```python
from build123d import *

# Parameters (mm, degrees)
BOSS_EXTRU_1_DEPTH = 150
CONG_1_R           = 15
BOSS_EXTRU_2_DEPTH = 2


with BuildPart() as part:
    # Esquisse1 → Boss.-Extru.1 (new body)
    with BuildSketch(Plane.XY):
        with BuildLine():
            Line((-112.5, 0), (112.5, 0))
            Line((112.5, 0), (112.5, 77.803254504))
            ThreePointArc((112.5, 77.803254504), (109.706079374, 82.982099708), (103.843702056, 83.490983093))
            Line((103.843702056, 83.490983093), (100.822174185, 82.206822173))
            Line((100.822174185, 82.206822173), (101.593849269, 84))
            Line((101.593849269, 84), (100.593849269, 84))
            Line((100.593849269, 84), (98.047294459, 81.066628108))
            Line((98.047294459, 81.066628108), (94.513975375, 79.668180307))
            Line((94.513975375, 79.668180307), (96.868414967, 84))
            Line((96.868414967, 84), (95.868414967, 84))
            Line((95.868414967, 84), (91.710401321, 78.600485349))
            Line((91.710401321, 78.600485349), (88.141932533, 77.29433432))
            Line((88.141932533, 77.29433432), (91.793248094, 84))
            Line((91.793248094, 84), (90.793248094, 84))
            Line((90.793248094, 84), (85.311557961, 76.299859694))
            Line((85.311557961, 76.299859694), (81.710349964, 75.086887739))
            Line((81.710349964, 75.086887739), (86.372418591, 84))
            Line((86.372418591, 84), (85.372418591, 84))
            Line((85.372418591, 84), (78.855086787, 74.166305212))
            Line((78.855086787, 74.166305212), (75.223572191, 73.047331693))
            Line((75.223572191, 73.047331693), (80.613241264, 84))
            Line((80.613241264, 84), (79.613241264, 84))
            Line((79.613241264, 84), (72.345349134, 72.201263116))
            Line((72.345349134, 72.201263116), (68.685981021, 71.177043896))
            Line((68.685981021, 71.177043896), (74.526463538, 84))
            Line((74.526463538, 84), (73.526463538, 84))
            Line((73.526463538, 84), (65.786742319, 70.406060788))
            Line((65.786742319, 70.406060788), (62.101992586, 69.477287727))
            Line((62.101992586, 69.477287727), (68.126397614, 84))
            Line((68.126397614, 84), (67.126397614, 84))
            Line((67.126397614, 84), (59.183696671, 68.781910885))
            Line((59.183696671, 68.781910885), (55.476054359, 67.949211366))
            Line((55.476054359, 67.949211366), (61.430986278, 84))
            Line((61.430986278, 84), (60.430986278, 84))
            Line((60.430986278, 84), (52.540672534, 67.329910517))
            Line((52.540672534, 67.329910517), (48.81264215, 66.593847028))
            Line((48.81264215, 66.593847028), (54.461792967, 84))
            Line((54.461792967, 84), (53.461792967, 84))
            Line((53.461792967, 84), (45.862157261, 66.051040507))
            Line((45.862157261, 66.051040507), (42.116257084, 65.412110258))
            Line((42.116257084, 65.412110258), (47.243908802, 84))
            Line((47.243908802, 84), (46.243908802, 84))
            Line((46.243908802, 84), (39.152662178, 64.946164731))
            Line((39.152662178, 64.946164731), (35.391422557, 64.404799318))
            Line((35.391422557, 64.404799318), (39.805772012, 84))
            Line((39.805772012, 84), (38.805772012, 84))
            Line((38.805772012, 84), (32.416719538, 64.01602953))
            Line((32.416719538, 64.01602953), (28.642681183, 63.572594644))
            Line((28.642681183, 63.572594644), (32.178898512, 84))
            Line((32.178898512, 84), (31.178898512, 84))
            Line((31.178898512, 84), (25.658879458, 63.261263209))
            Line((25.658879458, 63.261263209), (21.874591726, 62.91605839))
            Line((21.874591726, 62.91605839), (24.397526133, 84))
            Line((24.397526133, 84), (23.397526133, 84))
            Line((23.397526133, 84), (18.883706848, 62.682375611))
            Line((18.883706848, 62.682375611), (15.09172602, 62.435634044))
            Line((15.09172602, 62.435634044), (16.498178932, 84))
            Line((16.498178932, 84), (15.498178932, 84))
            Line((15.498178932, 84), (12.095778325, 62.279757774))
            Line((12.095778325, 62.279757774), (8.298665877, 62.131646133))
            Line((8.298665877, 62.131646133), (8.519161913, 84))
            Line((8.519161913, 84), (7.519161913, 84))
            Line((7.519161913, 84), (5.299679125, 62.053681665))
            Line((5.299679125, 62.053681665), (1.5, 62.004299999))
            Line((1.5, 62.004299999), (1, 84))
            Line((1, 84), (-1, 84))
            Line((-1, 84), (-1.5, 62.004299999))
            Line((-1.5, 62.004299999), (-5.299679125, 62.053681665))
            Line((-5.299679125, 62.053681665), (-7.519161913, 84))
            Line((-7.519161913, 84), (-8.519161913, 84))
            Line((-8.519161913, 84), (-8.298665877, 62.131646133))
            Line((-8.298665877, 62.131646133), (-12.095778325, 62.279757774))
            Line((-12.095778325, 62.279757774), (-15.498178932, 84))
            Line((-15.498178932, 84), (-16.498178932, 84))
            Line((-16.498178932, 84), (-15.09172602, 62.435634044))
            Line((-15.09172602, 62.435634044), (-18.883706848, 62.682375611))
            Line((-18.883706848, 62.682375611), (-23.397526133, 84))
            Line((-23.397526133, 84), (-24.397526133, 84))
            Line((-24.397526133, 84), (-21.874591726, 62.91605839))
            Line((-21.874591726, 62.91605839), (-25.658879458, 63.261263209))
            Line((-25.658879458, 63.261263209), (-31.178898512, 84))
            Line((-31.178898512, 84), (-32.178898512, 84))
            Line((-32.178898512, 84), (-28.642681183, 63.572594644))
            Line((-28.642681183, 63.572594644), (-32.416719538, 64.01602953))
            Line((-32.416719538, 64.01602953), (-38.805772012, 84))
            Line((-38.805772012, 84), (-39.805772012, 84))
            Line((-39.805772012, 84), (-35.391422557, 64.404799318))
            Line((-35.391422557, 64.404799318), (-39.152662178, 64.946164731))
            Line((-39.152662178, 64.946164731), (-46.243908802, 84))
            Line((-46.243908802, 84), (-47.243908802, 84))
            Line((-47.243908802, 84), (-42.116257084, 65.412110258))
            Line((-42.116257084, 65.412110258), (-45.862157261, 66.051040507))
            Line((-45.862157261, 66.051040507), (-53.461792967, 84))
            Line((-53.461792967, 84), (-54.461792967, 84))
            Line((-54.461792967, 84), (-48.81264215, 66.593847028))
            Line((-48.81264215, 66.593847028), (-52.540672534, 67.329910517))
            Line((-52.540672534, 67.329910517), (-60.430986278, 84))
            Line((-60.430986278, 84), (-61.430986278, 84))
            Line((-61.430986278, 84), (-55.476054359, 67.949211366))
            Line((-55.476054359, 67.949211366), (-59.183696671, 68.781910885))
            Line((-59.183696671, 68.781910885), (-67.126397614, 84))
            Line((-67.126397614, 84), (-68.126397614, 84))
            Line((-68.126397614, 84), (-62.101992586, 69.477287727))
            Line((-62.101992586, 69.477287727), (-65.786742319, 70.406060788))
            Line((-65.786742319, 70.406060788), (-73.526463538, 84))
            Line((-73.526463538, 84), (-74.526463538, 84))
            Line((-74.526463538, 84), (-68.685981021, 71.177043896))
            Line((-68.685981021, 71.177043896), (-72.345349134, 72.201263116))
            Line((-72.345349134, 72.201263116), (-79.613241264, 84))
            Line((-79.613241264, 84), (-80.613241264, 84))
            Line((-80.613241264, 84), (-75.223572191, 73.047331693))
            Line((-75.223572191, 73.047331693), (-78.855086787, 74.166305212))
            Line((-78.855086787, 74.166305212), (-85.372418591, 84))
            Line((-85.372418591, 84), (-86.372418591, 84))
            Line((-86.372418591, 84), (-81.710349964, 75.086887739))
            Line((-81.710349964, 75.086887739), (-85.311557961, 76.299859694))
            Line((-85.311557961, 76.299859694), (-90.793248094, 84))
            Line((-90.793248094, 84), (-91.793248094, 84))
            Line((-91.793248094, 84), (-88.141932533, 77.29433432))
            Line((-88.141932533, 77.29433432), (-91.710401321, 78.600485349))
            Line((-91.710401321, 78.600485349), (-95.868414967, 84))
            Line((-95.868414967, 84), (-96.868414967, 84))
            Line((-96.868414967, 84), (-94.513975375, 79.668180307))
            Line((-94.513975375, 79.668180307), (-98.047294459, 81.066628108))
            Line((-98.047294459, 81.066628108), (-100.593849269, 84))
            Line((-100.593849269, 84), (-101.593849269, 84))
            Line((-101.593849269, 84), (-100.822174185, 82.206822173))
            Line((-100.822174185, 82.206822173), (-103.843702056, 83.490983093))
            ThreePointArc((-103.843702056, 83.490983093), (-109.706079374, 82.982099708), (-112.5, 77.803254504))
            Line((-112.5, 77.803254504), (-112.5, 0))
        make_face()
    extrude(amount=BOSS_EXTRU_1_DEPTH)

    # Congé1
    cong_1_edges = [part.edges().sort_by_distance(p)[0] for p in [
        (112.5, 0, 75),
        (-112.5, 0, 75),
    ]]
    fillet(cong_1_edges, radius=CONG_1_R)

    # Esquisse2 → Boss.-Extru.2 (add)
    # profile 1 of 2: a face of its own
    with BuildSketch(Plane.XZ):
        Polygon((85, 134), (111, 150), (125, 150), (125, 102), (99, 86), (99, 64), (125, 48), (125, 0), (111, 0), (85, 16), (85, 34.748316978), align=None)
        with BuildLine():
            Line((120.5, 133), (120.5, 117))
            ThreePointArc((120.5, 117), (118.5, 115), (116.5, 117))
            Line((116.5, 117), (116.5, 133))
            ThreePointArc((116.5, 133), (118.5, 135), (120.5, 133))
        make_face(mode=Mode.SUBTRACT)
        with BuildLine():
            Line((120.5, 17), (120.5, 33))
            ThreePointArc((120.5, 33), (118.5, 35), (116.5, 33))
            Line((116.5, 33), (116.5, 17))
            ThreePointArc((116.5, 17), (118.5, 15), (120.5, 17))
        make_face(mode=Mode.SUBTRACT)
    # profile 2 of 2: a face of its own
    with BuildSketch(Plane.XZ):
        Polygon((-85, 34.748316978), (-85, 134), (-111, 150), (-125, 150), (-125, 102), (-99, 86), (-99, 64), (-125, 48), (-125, 0), (-111, 0), (-85, 16), align=None)
        with BuildLine():
            Line((-120.5, 133), (-120.5, 117))
            ThreePointArc((-120.5, 117), (-118.5, 115), (-116.5, 117))
            Line((-116.5, 117), (-116.5, 133))
            ThreePointArc((-116.5, 133), (-118.5, 135), (-120.5, 133))
        make_face(mode=Mode.SUBTRACT)
        with BuildLine():
            Line((-120.5, 17), (-120.5, 33))
            ThreePointArc((-120.5, 33), (-118.5, 35), (-116.5, 33))
            Line((-116.5, 33), (-116.5, 17))
            ThreePointArc((-116.5, 17), (-118.5, 15), (-120.5, 17))
        make_face(mode=Mode.SUBTRACT)
    extrude(amount=BOSS_EXTRU_2_DEPTH)


solid = part.part
```
The listing builds one solid part. Answer for the finished solid, in the listing's coordinates (mm). A direction names the side the tool comes from. Coordinates: 2 decimals unless noted, no trailing zeros. Write each loop counter-clockwise with the first axis right and the second up, starting at its lowest first coordinate (ties: lowest second). Pieces come first, ordered by that corner, then holes. Notation, with made-up numbers: (89.25, 13.5) - (93.25, 13.5) arc R11 cw to (93.25, 32.5) - close; hole circle Ø9 at (9, -35). An arc over 180 degrees is marked (long way). Return JSON: item names as keys, results as strings. Group by question number.
1. Determine the mould class of faces 1 (the flat face through (93.82, 81.34, 73.95)), 2 (the flat face through (-2, 33, 0)) for opening direction X: released by +X, released by -X, zero draft, split by the parting line, or undercut.
2. A cutting plane is placed at B-B, the plane y = 59.5. Determine the outline of the cut face in (x, z).
3. Which of the six approach directions +Z, -Z, +X, -X, +Y, -Y give full straight-line access (tool end or side, diameter ignored) to faces 3 (the flat face through (63.21, 76.5, 73.95)), 4 (the flat face through (96, -2, 76)), 5 (the flat face through (13.82, 73.29, 73.95)), 6 (the flat face through (-98, -1, 8))?
4. Straight lines are drawn through the part: L1, parallel to Y at x = 101.5, z = 14.5; L2, parallel to X at y = 60.5, z = 68; L3, parallel to Y at x = -92.5, z = 31.5. For each, find the intervals that lie inside material, in ascending order.
5. Given pin 1 (3 mm diameter, centred on x = -93.5, z = 104.5, fed in from +Y); pin 2 (5 mm diameter, centred on x = 33.5, z = 54.5, fed in from -Y); pin 3 (1.6 mm diameter, centred on y = -1, z = 73.5, fed in from -X), each flat-ended and moving along its own axis, determine where each tip first touches the part or whether it passes through.
6. A cutting plane is placed at A-A, the plane z = 27. Give the number of separate pieces and of enclosed holes in the cut face, plus the area to 3 significant figures.
Ans:
{
 "1": {"face 1": "undercut", "face 2": "zero draft"},
 "2": {"outline": "(-112.5, 0) - (112.5, 0) - (112.5, 150) - (-112.5, 150) - close"},
 "3": {"face 3": "+Z, -Z", "face 4": "+Z, -Z, +X, -X, -Y", "face 5": "+Z, -Z, +Y", "face 6": "-Z, -Y"},
 "4": {"L1": "-2 to 0, 0.54 to 82.49, 83.78 to 84", "L2": "-112.5 to 112.5", "L3": "-2 to 79.63"},
 "5": {"pin 1": "y = 82.87", "pin 2": "y = 0", "pin 3": "x = -99"},
 "6": {"separate pieces": "3", "enclosed holes": "0", "area": "16,700 mm²"}
}
